from build123d import *

# Parameters (mm, degrees)
F0_W     = 127
F0_H     = 44.45
F1_DEPTH = 6.35
F3_DEPTH = 6.35


with BuildPart() as f1:
    # F0 (on Top) → F1 (new body)
    with BuildSketch(Plane.XY):
        Rectangle(F0_W, F0_H)
    extrude(amount=F1_DEPTH)

    # F2 (on face) → F3 (cut, through all)
    with BuildSketch(Plane.XY.offset(6.35)):
        with BuildLine():
            ThreePointArc((-46.55, 0), (-50.8, 4.25), (-55.05, 0))
            Line((-55.05, 0), (-46.55, 0))
        make_face()
        with BuildLine():
            ThreePointArc((55.05, 0), (50.8, 4.25), (46.55, 0))
            Line((46.55, 0), (55.05, 0))
        make_face()
        with BuildLine():
            Line((55.05, 0), (46.55, 0))
            ThreePointArc((46.55, 0), (50.8, -4.25), (55.05, 0))
        make_face()
        with BuildLine():
            ThreePointArc((4.7625, 0), (0, 4.7625), (-4.7625, 0))
            Line((-4.7625, 0), (4.7625, 0))
        make_face()
        with BuildLine():
            Line((4.7625, 0), (-4.7625, 0))
            ThreePointArc((-4.7625, 0), (0, -4.7625), (4.7625, 0))
        make_face()
        with BuildLine():
            Line((-46.55, 0), (-55.05, 0))
            ThreePointArc((-55.05, 0), (-50.8, -4.25), (-46.55, 0))
        make_face()
    extrude(amount=-F3_DEPTH, mode=Mode.SUBTRACT)


solid = f1.part
Verification items for the finished model (mm, model axes). Coordinates: 2 decimals unless noted, no trailing zeros. Loops run counter-clockwise (first coordinate to the right, second up) from the corner with the lowest first, then second, coordinate; pieces in that order, holes last. Notation, with made-up numbers: (79, -21) -> (120, -21) arc R25 ccw to (120, -4) -> close; hole circle Ø7 at (85, 87). An arc over 180 degrees is marked (long way). Answer as CSV lines item,"result".
1) Thickness scan on L1, parallel to X at y = 0, z = 4.75; L2, parallel to Y at x = -50.8, z = 2.25 (3 decimals); L3, parallel to X at y = 3, z = 1. Record the ranges inside material, lowest first. Write a range as from..to.
Found:
L1,"x = -63.5..-55.05, -46.55..-4.76, 4.76..46.55, 55.05..63.5"
L2,"y = -22.225..-4.25, 4.25..22.225"
L3,"x = -63.5..-53.81, -47.79..-3.7, 3.7..47.79, 53.81..63.5"
2) Cross-section at B-B, the plane z = 5.25. Count the separate pieces of the cut face and the enclosed holes in it, then the cut area to 3 significant figures.
Found:
separate pieces,"1"
enclosed holes,"3"
area,"5,460 mm2"
3) Cross-section at C-C, the plane x = 50.8. Record the cut outline in (y, z) (3 decimals), then the cut area to 3 significant figures.
Found:
outline,"(-22.225, 0) -> (-4.25, 0) -> (-4.25, 6.35) -> (-22.225, 6.35) -> close; (4.25, 0) -> (22.225, 0) -> (22.225, 6.35) -> (4.25, 6.35) -> close"
area,"228 mm2"
4) Release check for a two-part mould opening along X. For faces 1 (the flat face through (-1, 5, 0)), 2 (the cylindrical face through (46.746, -1.277, 3.219)), 3 (the flat face through (63.5, 0, 3)), 4 (the flat face through (-63.5, 0, 3)) record: +X half, -X half, draft (parallel to the pull), parting line (faces both ways), or undercut.
Found:
face 1,"draft"
face 2,"undercut"
face 3,"+X half"
face 4,"-X half"
